Source: CAD feature listing. Evaluate the final solid. Frame: model axes, mm. A direction names the side the tool comes from. Give positions to 0.01 mm unless a question says otherwise; leave off trailing zeros. Order: outer loops, then holes, each group sorted by start corner. A loop starts at its lowest first (then second) coordinate and runs counter-clockwise, first axis right, second up. Notation, with made-up numbers: (5.5, 57) - (54.5, 57) arc R11 ccw to (54.5, 62) - close; hole circle Ø1 at (85, -28). An arc over 180 degrees is marked (long way). Use CSV: the item, a comma, the result in double quotes.
Autodesk Inventor part; units mm, degrees
ref_plane "YZ Plane" through (0, 0, 0) normal (1, 0, 0) x (0, 1, 0)
ref_plane "XZ Plane" through (0, 0, 0) normal (0, 1, 0) x (-1, 0, 0)
ref_plane "XY Plane" through (0, 0, 0) normal (0, 0, 1) x (1, 0, 0)
sketch "스케치4" plane through (0, 0, 0) normal (0, 0, 1) x (1, 0, 0)
  circle A0 centre (0, 0) radius 30
  dimension "d28" = 60
extrude "돌출4" add sketch "스케치4" along normal blind 9
sketch "스케치6" plane through (0, 0, 0) normal (0, 0, -1) x (-1, 0, 0)
  circle A0 centre (0, 0) radius 17.5
  dimension "d34" = 35
extrude "돌출6" add sketch "스케치6" along normal blind 6
sketch "스케치9" plane through (0, 0, -6) normal (0, 0, -1) x (-1, 0, 0)
  circle A0 centre (0, 0) radius 9.5
  dimension "d44" = 19
extrude "돌출9" cut sketch "스케치9" against normal blind 6
sketch "스케치12" plane through (0, 0, 9) normal (0, 0, 1) x (1, 0, 0)
  circle A0 centre (0, 24) radius 3
  point P0 (0, 0)
  dimension "d61" = 6
  dimension "d62" = 24
hole "구멍1" at (0, 24, 9) direction (0, 0, -1) diameter 3.4 end through all counterbore diameter 6 counterbore depth 3.3
sketch "스케치13" plane through (0, 0, 9) normal (0, 0, 1) x (1, 0, 0)
  circle A0 centre (0, 0) radius 15
  dimension "d74" = 30
extrude "돌출11" cut sketch "스케치13" against normal blind 5
sketch "스케치14" plane through (0, 0, 4) normal (0, 0, 1) x (1, 0, 0)
  circle A0 centre (0, 0) radius 4
  dimension "d77" = 8
extrude "돌출12" cut sketch "스케치14" against normal up to next
pattern_circular "원형 패턴3" count 4 over 360 about axis through (0, 0, 4) along (0, 0, -1) of "구멍1"
fillet "모깎기3" radius 3 2 edges at (-30, 0, 9) (9.5, 0, 0)
properties part number "도면2-3번"
Item 1: Section A-A on z = 0.75. Return the cut outline in (x, y), then the cut area to 3 significant figures.
Filled in:
outline,"circle Ø60 at (0, 0); hole circle Ø3.4 at (-24, 0); hole circle Ø8 at (0, 0); hole circle Ø3.4 at (0, -24); hole circle Ø3.4 at (0, 24); hole circle Ø3.4 at (24, 0)"
area,"2,740 mm2"
Item 2: Mould query, pull axis X, two halves, no side actions, for faces 1 (the flat face through (13, -13, 0)), 2 (the cylindrical face through (-0.65, -22.43, 2.81)), 3 (the cylindrical face through (-29.97, -1.32, 2.96)), 4 (the flat face through (-2, -24, 5.7)). Classes: released by +X, released by -X, zero draft, split by the parting line, or undercut.
Filled in:
face 1,"zero draft"
face 2,"undercut"
face 3,"split by the parting line"
face 4,"undercut"
Item 3: First-contact query: pin 1 (5.5 mm diameter, centred on x = 0, y = -24, fed in from -Z); pin 2 (4 mm diameter, centred on x = -21.5, z = 6, fed in from +Y); pin 3 (6 mm diameter, centred on x = 19.5, z = -2.5, fed in from +Y). Flat tips, straight axial feed; report the tip coordinate or a pass-through.
Filled in:
pin 1,"stops at z = 0"
pin 2,"stops at y = 22.8"
pin 3,"stops at y = 24.12"
Item 4: Set-up query: faces 5 (the cylindrical face through (-4.38, -8.43, -4.52)), 6 (the flat face through (-8, -8, -6)), 7 (the cylindrical face through (-14.985, 0.66, 6.535)). Return all of +Z, -Z, +X, -X, +Y, -Y with unobstructed straight access to the full face (end or side cutting, diameter ignored); none if empty.
Filled in:
face 5,"-Z"
face 6,"-Z, +X, -X, +Y, -Y"
face 7,"+Z"
Item 5: Material intervals for line 1 (Y direction, x = 0, z = 7.6); line 2 (Z direction, x = 15.5, y = -10); line 3 (Y direction, x = 0, z = 6.8), sorted ascending. Write a range as from..to.
Filled in:
line 1,"y = -29.54..-27, -21..-15, 15..21, 27..29.54"
line 2,"z = 0..9"
line 3,"y = -29.89..-27, -21..-15, 15..21, 27..29.89"
Item 6: Section D-D on z = 8. Return the cut outline in (x, y).
Filled in:
outline,"circle Ø58.47 at (0, 0); hole circle Ø6 at (-24, 0); hole circle Ø30 at (0, 0); hole circle Ø6 at (0, -24); hole circle Ø6 at (0, 24); hole circle Ø6 at (24, 0)"
Item 7: Section B-B on y = 0. Count the separate pieces of the cut face and the enclosed holes in it, then the cut area to 3 significant figures.
Filled in:
separate pieces,"4"
enclosed holes,"0"
area,"376 mm2"
